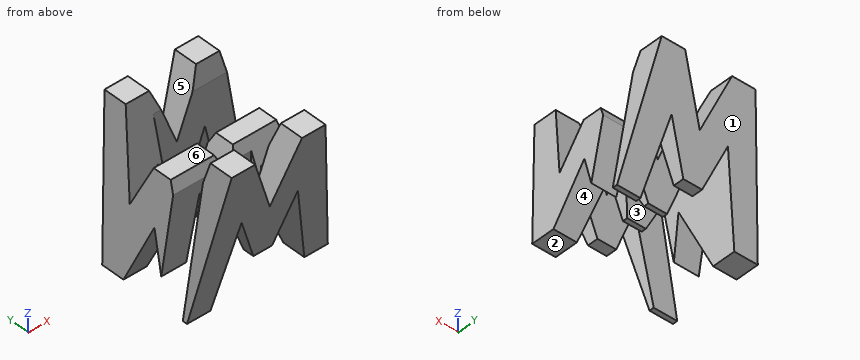
from build123d import *

# Parameters (mm, degrees)
F0_W     = 38.1
F0_H     = 38.1
F1_DEPTH = 38.1
F5_DEPTH = 38.1
F7_DEPTH = 38.1
F8_W     = 25.4
F8_H     = 7.62
F9_DEPTH = 38.1


with BuildPart() as f1:
    # F0 (on Front) → F1 (new body)
    with BuildSketch(Plane.XZ):
        with Locations((19.05, 19.05)):
            Rectangle(F0_W, F0_H)
    extrude(amount=F1_DEPTH)

    # F4 (on face) → F5 (cut)
    with BuildSketch(Plane.YZ.offset(38.1)):
        Polygon((-6.35, 38.1), (-31.75, 38.1), (-26.67, 16.814783), (-21.59, 28.575), (-16.51, 28.575), (-11.43, 17.16294), align=None)
        Polygon((-31.75, 0), (-38.1, 38.1), (-38.1, 0), align=None)
        Polygon((-19.05, 15.875), (-25.4, 0), (-12.7, 0), align=None)
        Polygon((0, 0), (0, 38.1), (-6.35, 0), align=None)
    extrude(amount=-F5_DEPTH, mode=Mode.SUBTRACT)

    # F6 (on offset) → F7 (cut)
    with BuildSketch(Plane.XZ.offset(38.1)):
        Polygon((0, 38.1), (0, 0), (6.35, 38.1), align=None)
        Polygon((11.43, 22.225), (6.35, 0), (31.75, 0), (26.67, 22.225), (21.59, 9.525), (16.51, 9.525), align=None)
        Polygon((25.4, 38.1), (12.7, 38.1), (19.05, 22.225), align=None)
        Polygon((31.75, 38.1), (38.1, 0), (38.1, 38.1), align=None)
    extrude(amount=-F7_DEPTH, mode=Mode.SUBTRACT)

    # F8 (on offset) → F9 (cut)
    with BuildSketch(Plane.XY.offset(38.1)):
        with Locations((25.4, -11.43)):
            Rectangle(F8_W, F8_H)
        with Locations((12.7, -26.67)):
            Rectangle(F8_W, F8_H)
    extrude(amount=-F9_DEPTH, mode=Mode.SUBTRACT)


solid = f1.part
Could you check a few things on this model? Use its own coordinates, in mm. Face numbers are marked on the shaded views. A direction names the side the tool comes from. Coordinates: 2 decimals unless noted, no trailing zeros. Order: outer loops, then holes, each group sorted by start corner. A loop starts at its lowest first (then second) coordinate and runs counter-clockwise, first axis right, second up. Notation, with made-up numbers: (-39, -33) -> (-29, -33) arc R31 cw to (-29, -6) -> close; hole circle Ø5 at (82, -14). An arc over 180 degrees is marked (long way). One line per item, written item: value. Start each with the question number.
1) Imagine slicing it at A-A on x = 3.5. List the corners of the cut face in (y, z) for me (3 decimals), plus the area to 3 significant figures.
2) Imagine slicing it at C-C on z = 24.5. Count the separate pieces of the cut face and the enclosed holes in it, plus the area to 3 significant figures.
3) I'm going to push flat-ended pins straight in: pin 1 (15.5 mm diameter, centred on x = 12, z = 19.5, fed in from -Y); pin 2 (3.5 mm diameter, centred on y = -29.5, z = 23.5, fed in from -X) (3 decimals); pin 3 (4 mm diameter, centred on x = 12, z = 19, fed in from +Y). Where does each tip first touch, or does it pass through?
4) Which directions (+Z, -Z, +X, -X, +Y, -Y) give clear straight access to the entire face, cutting with the end or side of a thin tool? Please do the marked faces 4, 5 and 6.
5) If I drill on L1, parallel to Y at x = 31, z = 9.5; L2, parallel to Y at x = 4, z = 19.5; L3, parallel to X at y = -20.5, z = 13, over which ranges is the centre line in solid material (lowest first)? Write a range as [from, to].
6) Imagine slicing it at B-B on z = 29.5. List the corners of the cut face in (x, y) for me, plus the area to 3 significant figures.
7) We'd pull the mould along Y, two halves only. Please class the marked faces 1, 2 and 3: +Y half, -Y half, draft (parallel to the pull), parting line (faces both ways), or undercut.
Answer list:
1. outline: (-35.25, 21) -> (-31.75, 0) -> (-30.48, 0) -> (-30.48, 21) -> close; (-22.86, 6.35) -> (-19.05, 15.875) -> (-12.7, 0) -> (-6.35, 0) -> (-2.85, 21) -> (-10.499, 21) -> (-11.43, 17.163) -> (-13.138, 21) -> (-22.86, 21) -> close
1. area: 349 mm2
2. separate pieces: 6
2. enclosed holes: 0
2. area: 559 mm2
3. pin 1: stops at y = -36.29
3. pin 2: stops at x = 3.675
3. pin 3: stops at y = -2.85
4. face 4: -Z, +X, -X
4. face 5: +Z, +Y, -Y
4. face 6: +Z, +X, -X
5. L1: y = [-33.33, -21.6], [-16.5, -15.24], [-7.62, -4.77]
5. L2: y = [-35, -30.48], [-22.86, -12.47], [-10.86, -3.1]
5. L3: x = [2.17, 9.32], [15.12, 22.98], [28.78, 35.93]
6. outline: (4.92, -36.67) -> (16.14, -36.67) -> (16.14, -30.48) -> (4.92, -30.48) -> close; (4.92, -8.44) -> (12.7, -8.44) -> (12.7, -7.62) -> (16.14, -7.62) -> (16.14, -1.43) -> (4.92, -1.43) -> close; (21.96, -36.67) -> (33.18, -36.67) -> (33.18, -29.7) -> (25.4, -29.7) -> (25.4, -30.48) -> (21.96, -30.48) -> close; (21.96, -7.62) -> (33.18, -7.62) -> (33.18, -1.43) -> (21.96, -1.43) -> close
6. area: 290 mm2
7. face 1: +Y half
7. face 2: draft
7. face 3: undercut
